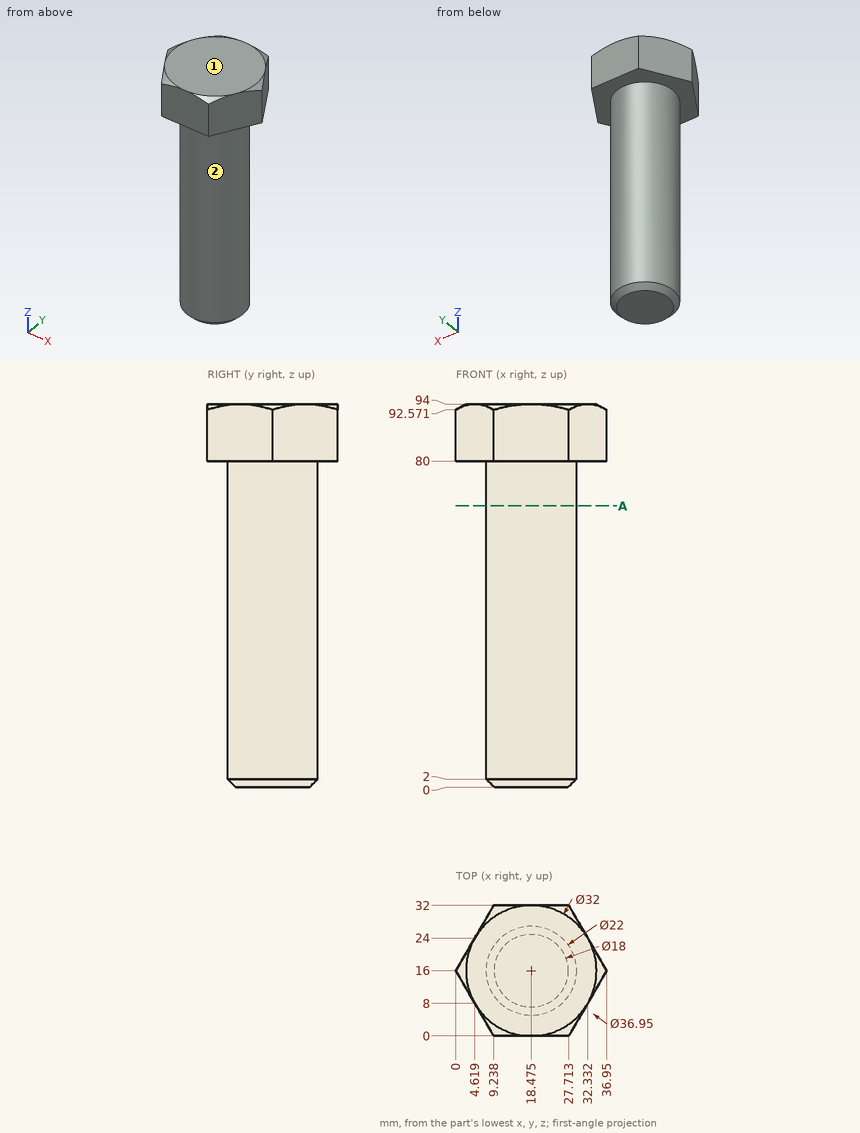
Study the drawing (mm; zero at the part's minimum x, y, z) and answer. A direction names the side the tool comes from. Give positions to 0.01 mm unless a question says otherwise; leave off trailing zeros. Write each loop counter-clockwise with the first axis right and the second up, starting at its lowest first coordinate (ties: lowest second). Pieces come first, ordered by that corner, then holes.
Item 1: Which of the six approach directions +Z, -Z, +X, -X, +Y, -Y give full straight-line access (tool end or side, diameter ignored) to the marked faces 1 and 2?
Item 2: Flat-ended cylindrical pins translate along their axes: P1, Ø6, axis at y = 20, z = 38, coming from the -X side; P2, Ø1, axis at y = 18.5, z = 52, coming from the +X side; P3, Ø12, axis at y = 9, z = 82.5, coming from the +X side. Find the tip coordinate at first contact, or state that the pin passes through.
Item 3: Section A-A, the plane z = 69 is taken. Write down the section's boundary in (x, y) (1 decimal), plus the area to 3 significant figures.
Item 4: Find the intervals of material crossed by line 1 along Z through (x, y) = (8.5, 3.5); line 2 along X through (y, z) = (8, 82); line 3 along Y through (x, z) = (18.5, 17), in increasing order.
Completed:
1. face 1: +Z, +X, -X, +Y, -Y
1. face 2: -Z
2. P1: stops at x = 7.52
2. P2: stops at x = 29.29
2. P3: stops at x = 36.37
3. outline: circle Ø22 at (18.5, 16)
3. area: 380 mm2
4. line 1: z = 80 to 94
4. line 2: x = 4.62 to 32.33
4. line 3: y = 5 to 27
